Source: CAD feature listing. Evaluate the final solid. Frame: model axes, mm. Round coordinates to 2 decimals unless told otherwise and drop trailing zeros. Order: outer loops, then holes, each group sorted by start corner. A loop starts at its lowest first (then second) coordinate and runs counter-clockwise, first axis right, second up. Notation, with made-up numbers: M 41,-29.5 L 50,-29.5 A19 cw 50,-18.5 Z; hole C 36,21 d8. An arc over 180 degrees is marked long. Answer in a Markdown table with one row per item. Add a question column.
```python
from build123d import *

# Parameters (mm, degrees)
ESBO_O1_W                = 360
ESBO_O1_H                = 320
ESBO_O1_R                = 11
ESBO_O1_R_2              = 37.5
ESBO_O1_R_3              = 30
ESBO_O1_R_4              = 22.5
RESSALTO_EXTRUS_O1_DEPTH = 5


with BuildPart() as part:
    # Esboço1 → Ressalto-extrusão1 (new body)
    with BuildSketch(Plane.XY):
        Rectangle(ESBO_O1_W, ESBO_O1_H)
        with Locations((0, 80)):
            Circle(ESBO_O1_R, mode=Mode.SUBTRACT)
        with Locations((-100, 80)):
            Circle(ESBO_O1_R, mode=Mode.SUBTRACT)
        with Locations((100, 80)):
            Circle(ESBO_O1_R, mode=Mode.SUBTRACT)
        with Locations((0, -60)):
            Circle(ESBO_O1_R, mode=Mode.SUBTRACT)
        with Locations((100, -60)):
            Circle(ESBO_O1_R, mode=Mode.SUBTRACT)
        with Locations((-100, -60)):
            Circle(ESBO_O1_R, mode=Mode.SUBTRACT)
        with Locations((-100, 0)):
            Circle(ESBO_O1_R_2, mode=Mode.SUBTRACT)
        Circle(ESBO_O1_R_2, mode=Mode.SUBTRACT)
        with Locations((100, 0)):
            Circle(ESBO_O1_R_2, mode=Mode.SUBTRACT)
        with Locations((100, -110)):
            Circle(ESBO_O1_R_3, mode=Mode.SUBTRACT)
        with Locations((0, -110)):
            Circle(ESBO_O1_R_3, mode=Mode.SUBTRACT)
        with Locations((-100, -110)):
            Circle(ESBO_O1_R_3, mode=Mode.SUBTRACT)
        with Locations((-100, 120)):
            Circle(ESBO_O1_R_4, mode=Mode.SUBTRACT)
        with Locations((0, 120)):
            Circle(ESBO_O1_R_4, mode=Mode.SUBTRACT)
        with Locations((100, 120)):
            Circle(ESBO_O1_R_4, mode=Mode.SUBTRACT)
    extrude(amount=RESSALTO_EXTRUS_O1_DEPTH)


solid = part.part
```
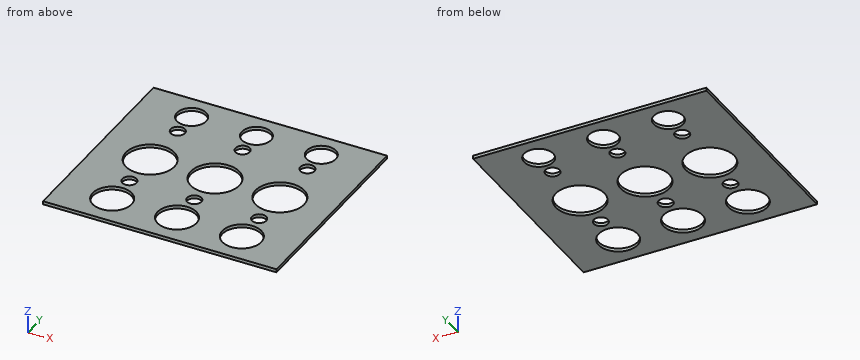
(1) Cut plane D-D (x = 18.5). Return loops of the section in (y, z), and give its area (3 significant figures).
(2) Cut plane C-C (z = 2.15). Count the separate pieces of the cut face and the enclosed holes in it, and give its area (3 significant figures).
(3) Pin query (flat end, axial travel): pin 1 (17.5 mm diameter, centred on x = 100, y = -60, fed in from -Z). Return the tip coordinate at first contact, or that it passes through.
(4) Cut plane B-B (x = 100). Return loops of the section in (y, z), and give its area (3 significant figures).
(5) Line query: line 1 (Y direction, x = -100, z = 2.8); line 2 (Y direction, x = -101.5, z = 4.6); line 3 (X direction, y = 80.5, z = 0.65). Output: solid intervals per line, ascending. Write a range as from..to.
(6) Cut plane A-A (y = 80). Return loops of the section in (x, z).
Answer list:
| question | item | result |
|---|---|---|
| 1 | outline | M -160,0 L -133.62,0 L -133.62,5 L -160,5 Z; M -86.38,0 L -32.62,0 L -32.62,5 L -86.38,5 Z; M 32.62,0 L 107.19,0 L 107.19,5 L 32.62,5 Z; M 132.81,0 L 160,0 L 160,5 L 132.81,5 Z |
| 1 | area | 910 mm² |
| 2 | separate pieces | 1 |
| 2 | enclosed holes | 15 |
| 2 | area | 86,400 mm² |
| 3 | pin 1 | through |
| 4 | outline | M -160,0 L -140,0 L -140,5 L -160,5 Z; M -80,0 L -71,0 L -71,5 L -80,5 Z; M -49,0 L -37.5,0 L -37.5,5 L -49,5 Z; M 37.5,0 L 69,0 L 69,5 L 37.5,5 Z; M 91,0 L 97.5,0 L 97.5,5 L 91,5 Z; M 142.5,0 L 160,0 L 160,5 L 142.5,5 Z |
| 4 | area | 480 mm² |
| 5 | line 1 | -160..-140, -80..-71, -49..-37.5, 37.5..69, 91..97.5, 142.5..160 |
| 5 | line 2 | -160..-139.96, -80.04..-70.9, -49.1..-37.47, 37.47..69.1, 90.9..97.55, 142.45..160 |
| 5 | line 3 | -180..-110.99, -89.01..-10.99, 10.99..89.01, 110.99..180 |
| 6 | outline | M -180,0 L -111,0 L -111,5 L -180,5 Z; M -89,0 L -11,0 L -11,5 L -89,5 Z; M 11,0 L 89,0 L 89,5 L 11,5 Z; M 111,0 L 180,0 L 180,5 L 111,5 Z |
